Design review of the part built by this model. Coordinates are the model's own, in mm. A direction names the side the tool comes from. Give positions to 0.01 mm unless a question says otherwise; leave off trailing zeros. Loops run counter-clockwise (first coordinate to the right, second up) from the corner with the lowest first, then second, coordinate; pieces in that order, holes last. Notation, with made-up numbers: M -6,38 L 30,38 A25 ccw 30,62 Z; hole C -5,15 d4. An arc over 180 degrees is marked long. Use one line per item in the form item = value. Start each with the question number.
from build123d import *

# Parameters (mm, degrees)
F0_R     = 25.15
F1_DEPTH = 4
F2_R     = 25.15
F2_R_2   = 22.5
F3_DEPTH = 22
F4_R     = 8
F5_DEPTH = 5
F6_R     = 4
F7_DEPTH = 25
F8_R     = 8
F9_DEPTH = 3


with BuildPart() as f1:
    # F0 (on Front) → F1 (new body)
    with BuildSketch(Plane.XZ):
        Circle(F0_R)
    extrude(amount=F1_DEPTH)

    # F2 (on face) → F3 (join)
    with BuildSketch(Plane.XZ.offset(4)):
        Circle(F2_R)
        Circle(F2_R_2, mode=Mode.SUBTRACT)
    extrude(amount=F3_DEPTH)

    # F4 (on face) → F5 (join)
    with BuildSketch(Plane.XZ.offset(4)):
        Circle(F4_R)
    extrude(amount=F5_DEPTH)

    # F6 (on face) → F7 (cut)
    with BuildSketch(Plane(origin=(0, 0, 0), x_dir=(-1, 0, 0), z_dir=(0, 1, 0))):
        Circle(F6_R)
    extrude(amount=-F7_DEPTH, mode=Mode.SUBTRACT)

    # F8 (on face) → F9 (cut)
    with BuildSketch(Plane(origin=(0, 0, 0), x_dir=(-1, 0, 0), z_dir=(0, 1, 0))):
        Circle(F8_R)
    extrude(amount=-F9_DEPTH, mode=Mode.SUBTRACT)


solid = f1.part
Q1. Wall thickness on probe 1 along Z at (x, y) = (0, -6.5); probe 2 along Z at (x, y) = (0, -18.25); probe 3 along Y at (x, z) = (-15.5, -6.5): over which ranges is each line inside the solid? List them lowest first.
Q2. The part is to be moulded in two halves that separate along X. For faces 1 (the cylindrical face through (-25.126, -12.818, 1.106)), 2 (the flat face through (10, -4, 0)), 3 (the flat face through (-6, 0, 6)), say which applies: pulls with the +X half, pulls with the -X half, needs draft (parallel to the pull), parting line crosses it, or undercut.
Q3. Take a section at D-D on z = -15.5. Give the boundary of the cut face in (x, y).
Q4. Take a section at A-A on z = 0. Give the boundary of the cut face in (x, y).
Q5. For faces 4 (the flat face through (-19, -26, -13)), 5 (the flat face through (4, -3, -2)), 6 (the cylindrical face through (10.382, -14.846, -19.961)), list the 3-axis set-ups (+Z, -Z, +X, -X, +Y, -Y) from which the entire face can be reached by the end or side of a thin tool; tool diameter is ignored.
Q6. Take a section at C-C on x = -15. Give the boundary of the cut face in (y, z).
Q7. Clearance check with flat-ended pins moving along their axes: pin 1 Ø4 at (x, y) = (-8, -5.5) entering from -Z; pin 2 Ø3 at (y, z) = (-13.5, 2) entering from +X (3 decimals); pin 3 Ø8 at (y, z) = (-8, 18.5) entering from +X. State where each tip first meets the part, or that it passes through.
Q8. Take a section at B-B on x = 0. Give the boundary of the cut face in (y, z).
Response values:
q1.probe_1 = -25.15 to -22.5, -8 to -4, 4 to 8, 22.5 to 25.15
q1.probe_2 = -25.15 to -22.5, 22.5 to 25.15
q1.probe_3 = -4 to 0
q2.face_1 = parting line crosses it
q2.face_2 = undercut
q2.face_3 = needs draft
q3.outline = M -19.81,-26 L -16.31,-26 L -16.31,-4 L 16.31,-4 L 16.31,-26 L 19.81,-26 L 19.81,0 L -19.81,0 Z
q4.outline = M -25.15,-26 L -22.5,-26 L -22.5,-4 L -8,-4 L -8,-9 L -4,-9 L -4,-3 L -8,-3 L -8,0 L -25.15,0 Z; M 4,-9 L 8,-9 L 8,-4 L 22.5,-4 L 22.5,-26 L 25.15,-26 L 25.15,0 L 8,0 L 8,-3 L 4,-3 Z
q5.face_4 = +Z, -Z, +X, -X, -Y
q5.face_5 = +Y
q5.face_6 = -Y
q6.outline = M -26,-20.19 L 0,-20.19 L 0,20.19 L -26,20.19 L -26,16.77 L -4,16.77 L -4,-16.77 L -26,-16.77 Z
q7.pin_1 = -24.42
q7.pin_2 = 25.145
q7.pin_3 = 20.55
q8.outline = M -26,-25.15 L 0,-25.15 L 0,-8 L -3,-8 L -3,-4 L -9,-4 L -9,-8 L -4,-8 L -4,-22.5 L -26,-22.5 Z; M -26,22.5 L -4,22.5 L -4,8 L -9,8 L -9,4 L -3,4 L -3,8 L 0,8 L 0,25.15 L -26,25.15 Z
